Build history of the part. All positions in model axes, mm. A direction names the side the tool comes from. Round coordinates to 2 decimals unless told otherwise and drop trailing zeros. Loops run counter-clockwise (first coordinate to the right, second up) from the corner with the lowest first, then second, coordinate; pieces in that order, holes last.
from build123d import *

# Parameters (mm, degrees)
SKETCH_1_W          = 80
SKETCH_1_H          = 56
EXTRUDE_1_DEPTH     = 200
CUT_EXTRUDE_1_DEPTH = 50
SKETCH_3_R          = 3.5
SKETCH_3_R_2        = 13
CUT_EXTRUDE_2_DEPTH = 10
SKETCH_4_R          = 2
SKETCH_4_W          = 27
SKETCH_4_H          = 36
CUT_EXTRUDE_3_DEPTH = 10
SKETCH_5_R          = 3
CUT_EXTRUDE_4_DEPTH = 10
SKETCH_6_R          = 3.500000002
SKETCH_6_R_2        = 3.5
CUT_EXTRUDE_5_DEPTH = 10
SKETCH_7_R          = 1.5
CUT_EXTRUDE_6_DEPTH = 10
SKETCH_8_W          = 165
SKETCH_8_H          = 50
CUT_EXTRUDE_7_DEPTH = 81


with BuildPart() as part:
    # 草图1 → 凸台-拉伸1 (new body)
    with BuildSketch(Plane.XY):
        Rectangle(SKETCH_1_W, SKETCH_1_H)
    extrude(amount=-EXTRUDE_1_DEPTH)

    # 草图2 → 切除-拉伸1 (cut)
    with BuildSketch(Plane(origin=(0, 28, 0), x_dir=(1, 0, 0), z_dir=(0, 1, 0))):
        with BuildLine():
            ThreePointArc((-34, 191), (-33.121320344, 193.121320344), (-31, 194))
            Line((-31, 194), (31, 194))
            ThreePointArc((31, 194), (33.121320344, 193.121320344), (34, 191))
            Line((34, 191), (34, 9))
            ThreePointArc((34, 9), (33.121320344, 6.878679656), (31, 6))
            Line((31, 6), (-31, 6))
            ThreePointArc((-31, 6), (-33.121320344, 6.878679656), (-34, 9))
            Line((-34, 9), (-34, 191))
        make_face()
    extrude(amount=-CUT_EXTRUDE_1_DEPTH, mode=Mode.SUBTRACT)

    # 草图3 → 切除-拉伸2 (cut)
    with BuildSketch(Plane.XY):
        with Locations((-28, 0)):
            Circle(SKETCH_3_R)
        Circle(SKETCH_3_R_2)
        with Locations((28, 0)):
            Circle(SKETCH_3_R)
    extrude(amount=-CUT_EXTRUDE_2_DEPTH, mode=Mode.SUBTRACT)

    # 草图4 → 切除-拉伸3 (cut)
    with BuildSketch(Plane.ZY.offset(40)):
        with Locations((-121.5, -5)):
            Circle(SKETCH_4_R)
        with Locations((-121.5, 19)):
            Circle(SKETCH_4_R)
        with Locations((-158.5, 19)):
            Circle(SKETCH_4_R)
        with Locations((-158.5, -5)):
            Circle(SKETCH_4_R)
        with Locations((-140, 7)):
            Rectangle(SKETCH_4_W, SKETCH_4_H)
    extrude(amount=-CUT_EXTRUDE_3_DEPTH, mode=Mode.SUBTRACT)

    # 草图5 → 切除-拉伸4 (cut)
    with BuildSketch(Plane(origin=(0, 0, -200), x_dir=(-1, 0, 0), z_dir=(0, 0, -1))):
        with Locations((24, 0)):
            Circle(SKETCH_5_R)
        with Locations((-24, 0)):
            Circle(SKETCH_5_R)
    extrude(amount=-CUT_EXTRUDE_4_DEPTH, mode=Mode.SUBTRACT)

    # 草图6 → 切除-拉伸5 (cut)
    with BuildSketch(Plane(origin=(0, -22, 0), x_dir=(1, 0, 0), z_dir=(0, 1, 0))):
        with Locations((-16, 166)):
            Circle(SKETCH_6_R)
        with Locations((-16, 113)):
            Circle(SKETCH_6_R_2)
    extrude(amount=-CUT_EXTRUDE_5_DEPTH, mode=Mode.SUBTRACT)

    # 草图7 → 切除-拉伸6 (cut)
    with BuildSketch(Plane(origin=(0, 28, 0), x_dir=(1, 0, 0), z_dir=(0, 1, 0))):
        with Locations((-37, 150)):
            Circle(SKETCH_7_R)
        with Locations((-37, 50)):
            Circle(SKETCH_7_R)
        with Locations((37, 50)):
            Circle(SKETCH_7_R)
        with Locations((37, 150)):
            Circle(SKETCH_7_R)
        with Locations((0, 197)):
            Circle(SKETCH_7_R)
        with Locations((0, 3)):
            Circle(SKETCH_7_R)
    extrude(amount=-CUT_EXTRUDE_6_DEPTH, mode=Mode.SUBTRACT)

    # 草图8 → 切除-拉伸7 (cut, through all)
    with BuildSketch(Plane(origin=(40, 0, 0), x_dir=(0, 0, -1), z_dir=(1, 0, 0))):
        with Locations((102.5, 3)):
            Rectangle(SKETCH_8_W, SKETCH_8_H)
    extrude(amount=-CUT_EXTRUDE_7_DEPTH, mode=Mode.SUBTRACT)


solid = part.part
(1) Slice it at C-C on y = -8. List the corners of the cut face in (x, z).
Responses:
outline: (-40, -200) - (40, -200) - (40, -185) - (34, -185) - (34, -191) arc R3 cw to (31, -194) - (-31, -194) arc R3 cw to (-34, -191) - (-34, -185) - (-40, -185) - close; (-40, -20) - (-34, -20) - (-34, -9) arc R3 cw to (-31, -6) - (-10.25, -6) - (-10.25, 0) - (-40, 0) - close; (10.25, -6) - (31, -6) arc R3 cw to (34, -9) - (34, -20) - (40, -20) - (40, 0) - (10.25, 0) - close
(2) Slice it at B-B on z = -113. List the corners of the cut face in (x, y).
Responses:
outline: (-40, -28) - (-19.5, -28) - (-19.5, -22) - (-40, -22) - close; (-12.5, -28) - (40, -28) - (40, -22) - (-12.5, -22) - close
(3) Slice it at D-D on y = 0. Count the separate pieces of the cut face and the enclosed holes in it, plus the area to 3 significant figures.
Responses:
separate pieces: 7
enclosed holes: 0
area: 932 mm2
(4) Pull direction Z, two halves, no side cores. Call faces 4 (the face through (-1, -28, -99)), 5 (the face through (-16.759, -24.958, -162.583)), 6 (the face through (-9, 13, 0)), 7 (the face through (-34, 3, -188)): +Z half, -Z half, draft (parallel to the pull), parting line (faces both ways), or undercut.
Responses:
face 4: draft
face 5: undercut
face 6: +Z half
face 7: undercut
(5) Pin check, flat tips, straight feed: P1, Ø5, axis at x = -1.5, z = -95, coming from the +Y side; P2, Ø4, axis at x = -28, y = 0, coming from the +Z side; P3, Ø0.9, axis at x = 0, z = -196.5, coming from the +Y side. Stop position of each tip, or through.
Responses:
P1: stops at y = -22
P2: stops at z = -194
P3: stops at y = 18
(6) Probe line 1 (Z direction, x = -26, y = 24.5); line 2 (Z direction, x = 0, y = 24); line 3 (Y direction, x = 0, z = -2). List the from-to ranges inside material, lowest first.
Responses:
line 1: z = -200 to -194, -6 to 0
line 2: z = -200 to -198.5, -195.5 to -194, -6 to -4.5, -1.5 to 0
line 3: y = -28 to -13, 13 to 18
(7) Which spindle directions (+Z, -Z, +X, -X, +Y, -Y) get a long thin tool onto all of the face, cutting with end or side? Do faces 1 (the face through (0, 3, -194)), 2 (the face through (-21, 0, -197)), 3 (the face through (-37, 3, -20)). Say none if no direction does.
Responses:
face 1: +Y
face 2: -Z
face 3: +X, -X, +Y
(8) Slice it at A-A on x = -16. List the corners of the cut face in (y, z), plus the area to 3 significant figures.
Responses:
outline: (-28, -200) - (28, -200) - (28, -194) - (-22, -194) - (-22, -169.5) - (-28, -169.5) - close; (-28, -162.5) - (-22, -162.5) - (-22, -116.5) - (-28, -116.5) - close; (-28, -109.5) - (-22, -109.5) - (-22, -6) - (28, -6) - (28, 0) - (-28, 0) - close
area: 1,720 mm2
